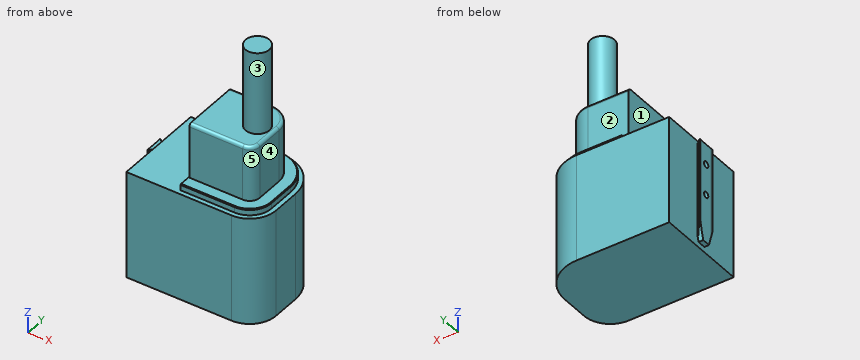
```python
from build123d import *

# Parameters (mm, degrees)
SKETCH1_W           = 85
SKETCH1_H           = 60
BOSS_EXTRUDE1_DEPTH = 69.5
BOSS_EXTRUDE2_DEPTH = 66.05
SKETCH3_W           = 3.16
SKETCH3_H           = 1.25
CUT_EXTRUDE1_DEPTH  = 103.54309143
CUT_EXTRUDE2_DEPTH  = 114.821131606
CUT_EXTRUDE3_DEPTH  = 89.402972801
BOSS_EXTRUDE3_DEPTH = 4
CHAMFER1_SIZE       = 0.5
BOSS_EXTRUDE4_DEPTH = 35.5
SKETCH8_R           = 7.75
BOSS_EXTRUDE5_DEPTH = 53.3
FILLET1_R           = 2
SKETCH9_R           = 2
CUT_EXTRUDE4_DEPTH  = 10


with BuildPart() as part:
    # Sketch1 → Boss-Extrude1 (new body)
    with BuildSketch(Plane.XY):
        Rectangle(SKETCH1_W, SKETCH1_H)
    extrude(amount=BOSS_EXTRUDE1_DEPTH)

    # Sketch2 → Boss-Extrude2 (add)
    with BuildSketch(Plane.XY.offset(69.5)):
        Polygon((-42.5, 3.495), (-42.79, 3.495), (-45.03, 5.73), (-45.66, 5.73), (-45.66, 4.45), (-45.533118158, 4.45), (-45.533118158, -4.45), (-45.66, -4.45), (-45.66, -5.73), (-45.03, -5.73), (-42.79, -3.495), (-42.5, -3.495), align=None)
    extrude(amount=-BOSS_EXTRUDE2_DEPTH)

    # Sketch3 → Cut-Extrude1 (cut, through all)
    with BuildSketch(Plane.XZ.offset(30)):
        with Locations((-44.08, 68.875)):
            Rectangle(SKETCH3_W, SKETCH3_H)
    extrude(amount=-CUT_EXTRUDE1_DEPTH, mode=Mode.SUBTRACT)

    # Sketch4 → Cut-Extrude2 (cut, through all)
    with BuildSketch(Plane.ZY.offset(42.5)):
        Polygon((3.45, 2.7), (14.31, 5.73), (3.45, 5.73), align=None)
        Polygon((3.45, -5.73), (3.45, -2.7), (14.31, -5.73), align=None)
    extrude(amount=CUT_EXTRUDE2_DEPTH, mode=Mode.SUBTRACT)

    # Sketch5 → Cut-Extrude3 (cut, through all)
    with BuildSketch(Plane.XY.offset(69.5)):
        with BuildLine():
            Line((42.5, -13), (42.5, -30))
            Line((42.5, -30), (25.5, -30))
            ThreePointArc((25.5, -30), (37.52081528, -25.02081528), (42.5, -13))
        make_face()
        with BuildLine():
            Line((17.5, 30), (42.5, 30))
            Line((42.5, 30), (42.5, 5))
            ThreePointArc((42.5, 5), (35.17766953, 22.67766953), (17.5, 30))
        make_face()
    extrude(amount=-CUT_EXTRUDE3_DEPTH, mode=Mode.SUBTRACT)

    # Sketch6 → Boss-Extrude3 (add)
    with BuildSketch(Plane.XY.offset(69.5)):
        with BuildLine():
            Line((17.5, 27), (-9.5, 27))
            Line((-9.5, 27), (-9.5, -27))
            Line((-9.5, -27), (17.308513795, -27))
            Line((17.308513795, -27), (25.5, -27))
            ThreePointArc((25.5, -27), (35.399494937, -22.899494937), (39.5, -13))
            Line((39.5, -13), (39.5, 5))
            ThreePointArc((39.5, 5), (33.056349186, 20.556349186), (17.5, 27))
        make_face()
    extrude(amount=BOSS_EXTRUDE3_DEPTH)

    # Chamfer1
    chamfer1_edges = [part.edges().sort_by_distance(p)[0] for p in [
        (33.056349186, 20.556349186, 73.5),
        (4, 27, 73.5),
        (8, -27, 73.5),
        (35.399494937, -22.899494937, 73.5),
        (39.5, -4, 73.5),
    ]]
    chamfer(chamfer1_edges, length=CHAMFER1_SIZE)

    # Sketch7 → Boss-Extrude4 (add)
    with BuildSketch(Plane.XY.offset(73.5)):
        with BuildLine():
            Line((-9, 19.5), (-9, -19.5))
            Line((-9, -19.5), (25.5, -19.5))
            ThreePointArc((25.5, -19.5), (30.096194078, -17.596194078), (32, -13))
            Line((32, -13), (32, 5))
            ThreePointArc((32, 5), (27.753048327, 15.253048327), (17.5, 19.5))
            Line((17.5, 19.5), (-9, 19.5))
        make_face()
    extrude(amount=BOSS_EXTRUDE4_DEPTH)

    # Sketch8 → Boss-Extrude5 (add)
    with BuildSketch(Plane.XY.offset(109)):
        with Locations((21.5, 0)):
            Circle(SKETCH8_R)
    extrude(amount=BOSS_EXTRUDE5_DEPTH)

    # Fillet1
    fillet1_edges = [part.edges().sort_by_distance(p)[0] for p in [
        (4.25, 19.5, 109),
        (8.25, -19.5, 109),
        (30.096194078, -17.596194078, 109),
        (32, -4, 109),
        (27.753048327, 15.253048327, 109),
    ]]
    fillet(fillet1_edges, radius=FILLET1_R)

    # Sketch9 → Cut-Extrude4 (cut)
    with BuildSketch(Plane.ZY.offset(45.533118158)):
        with Locations((55, 0)):
            Circle(SKETCH9_R)
        with Locations((35, 0)):
            Circle(SKETCH9_R)
    extrude(amount=-CUT_EXTRUDE4_DEPTH, mode=Mode.SUBTRACT)


solid = part.part
```
Part model, mm, in its own coordinate system. Face numbers are marked on the shaded views. A direction names the side the tool comes from. Coordinates: 2 decimals unless noted, no trailing zeros. Order: outer loops, then holes, each group sorted by start corner. A loop starts at its lowest first (then second) coordinate and runs counter-clockwise, first axis right, second up. Notation, with made-up numbers: (62.25, 45) -> (94.25, 45) arc R32 cw to (94.25, 80) -> close; hole circle Ø6 at (87.25, 23). An arc over 180 degrees is marked (long way). Put each result on its own line as item: value. Start each with the question number.
(1) Band-saw the part on B-B (z = 40). Give the cut face in (x, y) (3 decimals).
(2) Band-saw the part on C-C (x = 8.5). Give the cut face in (y, z), then the cut area to 3 significant figures.
(3) Pin check, flat tips, straight feed: pin 1 Ø14.5 at (x, y) = (4, 10) entering from +Z; pin 2 Ø4.5 at (y, z) = (-6, 72.5) entering from -X; pin 3 Ø5.5 at (y, z) = (-8, 88) entering from +X. Stop position of each tip, or through.
(4) Probe line 1 along Y through (x, z) = (-41.5, 35); line 2 along Z through (x, y) = (23, 21); line 3 along X through (y, z) = (5, 47). List the from-to ranges inside material, lowest first. Write a range as [from, to].
(5) Which spindle directions (+Z, -Z, +X, -X, +Y, -Y) get a long thin tool onto all of the face, cutting with end or side? Do the marked faces 1, 2, 3, 4 and 5. Say none if no direction does.
(6) Band-saw the part on D-D (z = 87). Give the cut face in (x, y), then the cut area to 3 significant figures.
Determined:
1. outline: (-45.66, -5.73) -> (-45.03, -5.73) -> (-42.79, -3.495) -> (-42.5, -3.495) -> (-42.5, -30) -> (25.5, -30) arc R17 ccw to (42.5, -13) -> (42.5, 5) arc R25 ccw to (17.5, 30) -> (-42.5, 30) -> (-42.5, 3.495) -> (-42.79, 3.495) -> (-45.03, 5.73) -> (-45.66, 5.73) -> (-45.66, 4.45) -> (-45.533, 4.45) -> (-45.533, -4.45) -> (-45.66, -4.45) -> close
2. outline: (-30, 0) -> (30, 0) -> (30, 69.5) -> (27, 69.5) -> (27, 73) -> (26.5, 73.5) -> (19.5, 73.5) -> (19.5, 107) arc R2 ccw to (17.5, 109) -> (-17.5, 109) arc R2 ccw to (-19.5, 107) -> (-19.5, 73.5) -> (-26.5, 73.5) -> (-27, 73) -> (-27, 69.5) -> (-30, 69.5) -> close
2. area: 5,770 mm²
3. pin 1: stops at z = 109
3. pin 2: stops at x = -9.5
3. pin 3: stops at x = 32
4. line 1: y = [-30, -2], [2, 30]
4. line 2: z = [0, 73.5]
4. line 3: x = [-45.66, -44.3], [-42.5, 42.5]
5. face 1: +Z, -X, +Y, -Y
5. face 2: +Z, +X, -X, +Y
5. face 3: +Z
5. face 4: +Z, +X, +Y, -Y
5. face 5: +Z, +X, -Y
6. outline: (-9, -19.5) -> (25.5, -19.5) arc R6.5 ccw to (32, -13) -> (32, 5) arc R14.5 ccw to (17.5, 19.5) -> (-9, 19.5) -> close
6. area: 1,540 mm²
